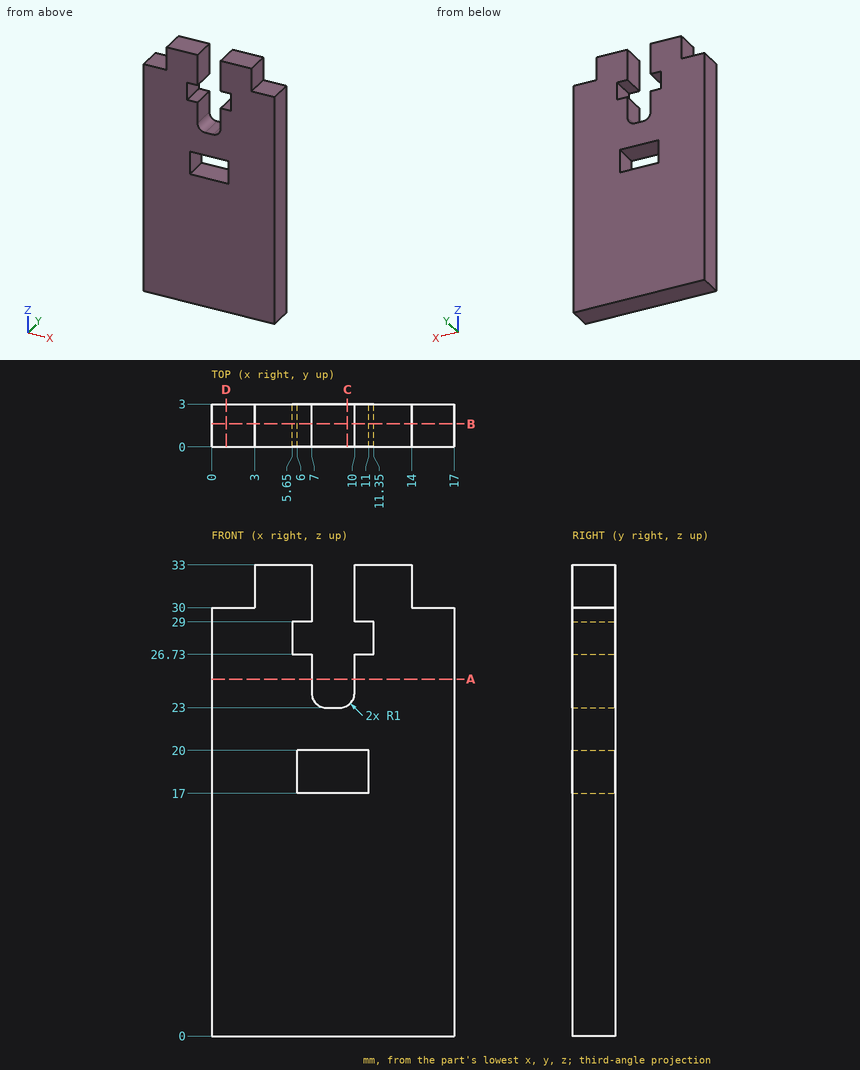
Answer from the drawing. Dimensions are ordinates in mm from the lowest x, y and z of the part. Give positions to 0.01 mm unless a question says otherwise; leave off trailing zeros. Write each loop counter-clockwise with the first axis right and the second up, starting at its lowest first coordinate (ties: lowest second). Pieces come first, ordered by that corner, then holes.
1) Section A-A (z = 25) is taken. Write down the section's boundary in (x, y).
2) Given P1, Ø0.9, axis at y = 2, z = 32, coming from the -X side; P2, Ø0.9, axis at x = 1.5, y = 1, coming from the +Z side; P3, Ø0.9, axis at y = 1, z = 31.5, coming from the +X side, each flat-ended and moving along its own axis, determine where each tip first touches the part or whether it passes through.
3) Section C-C (x = 9.5) is taken. Write down the section's boundary in (y, z), and give its area (3 significant figures).
4) Find the intervals of material crossed by L1, parallel to Z at x = 10.5, y = 0.4; L2, parallel to X at y = 1.25, z = 24.5; L3, parallel to Z at x = 5.75, y = 2.8, in increasing order.
5) Section B-B (y = 1.6) is taken. Write down the section's boundary in (x, z).
6) Section D-D (x = 1) is taken. Write down the section's boundary in (y, z).
Response:
1. outline: (0, 0) - (7, 0) - (7, 3) - (0, 3) - close; (10, 0) - (17, 0) - (17, 3) - (10, 3) - close
2. P1: stops at x = 3
2. P2: stops at z = 30
2. P3: stops at x = 14
3. outline: (0, 0) - (3, 0) - (3, 17) - (0, 17) - close; (0, 20) - (3, 20) - (3, 23.13) - (0, 23.13) - close
3. area: 60.4 mm2
4. L1: z = 0 to 17, 20 to 26.73, 29 to 33
4. L2: x = 0 to 7, 10 to 17
4. L3: z = 0 to 26.73, 29 to 33
5. outline: (0, 0) - (17, 0) - (17, 30) - (14, 30) - (14, 33) - (10, 33) - (10, 29) - (11.35, 29) - (11.35, 26.73) - (10, 26.73) - (10, 24) arc R1 cw to (9, 23) - (8, 23) arc R1 cw to (7, 24) - (7, 26.73) - (5.65, 26.73) - (5.65, 29) - (7, 29) - (7, 33) - (3, 33) - (3, 30) - (0, 30) - close; hole (6, 17) - (11, 17) - (11, 20) - (6, 20) - close
6. outline: (0, 0) - (3, 0) - (3, 30) - (0, 30) - close
